Part model, mm, in its own coordinate system. Round coordinates to 2 decimals unless told otherwise and drop trailing zeros. Loops run counter-clockwise (first coordinate to the right, second up) from the corner with the lowest first, then second, coordinate; pieces in that order, holes last. Notation, with made-up numbers: M 3.5,-3 L 47.5,-3 A36 cw 47.5,36 Z; hole C 52,85.25 d10. An arc over 180 degrees is marked long. Put each result on its own line as item: value. Start each with the question number.
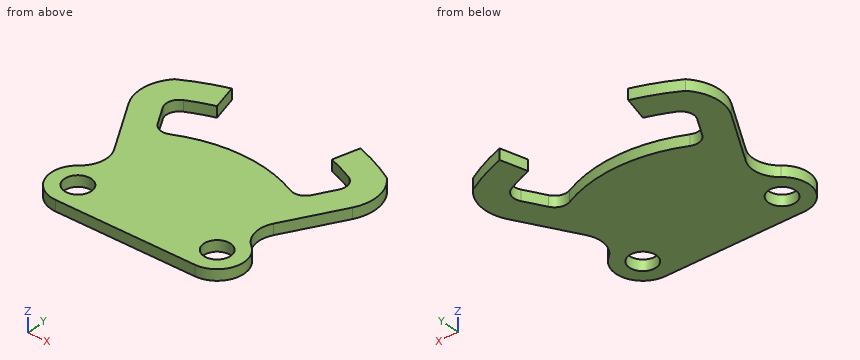
```python
from build123d import *

# Parameters (mm, degrees)
CROQUIS1_R              = 12.5
SALIENTE_EXTRUIR3_DEPTH = 10


with BuildPart() as part:
    # Croquis1 → Saliente-Extruir3 (new body)
    with BuildSketch(Plane.XY):
        with BuildLine():
            Line((-65, 0), (65, 0))
            ThreePointArc((65, 0), (88.615469852, 16.795758191), (80.499762007, 44.615233308))
            ThreePointArc((80.499762007, 44.615233308), (71.445806296, 59.527813514), (74.34888892, 76.730466615))
            Line((74.34888892, 76.730466615), (104.34888892, 128.691990842))
            ThreePointArc((104.34888892, 128.691990842), (109.189179993, 152.050160185), (99.153741511, 173.690919579))
            ThreePointArc((99.153741511, 173.690919579), (80.034708306, 183.287875939), (60, 190.787840283))
            Line((60, 190.787840283), (53.522714622, 166.614282159))
            ThreePointArc((53.522714622, 166.614282159), (65.481747035, 162.287217011), (77.094946128, 157.103053062))
            ThreePointArc((77.094946128, 157.103053062), (83.288324785, 149.82485993), (82.200740382, 140.330272281))
            Line((82.200740382, 140.330272281), (71.673300788, 122.09621203))
            ThreePointArc((71.673300788, 122.09621203), (64.832856812, 116.63391364), (56.102320229, 117.271180027))
            ThreePointArc((56.102320229, 117.271180027), (0, 130), (-56.102320229, 117.271180027))
            ThreePointArc((-56.102320229, 117.271180027), (-64.832856812, 116.63391364), (-71.673300788, 122.09621203))
            Line((-71.673300788, 122.09621203), (-82.200740382, 140.330272281))
            ThreePointArc((-82.200740382, 140.330272281), (-83.288324785, 149.82485993), (-77.094946128, 157.103053062))
            ThreePointArc((-77.094946128, 157.103053062), (-65.481747035, 162.287217011), (-53.522714622, 166.614282159))
            Line((-53.522714622, 166.614282159), (-60, 190.787840283))
            ThreePointArc((-60, 190.787840283), (-80.034708306, 183.287875939), (-99.153741511, 173.690919579))
            ThreePointArc((-99.153741511, 173.690919579), (-109.189179993, 152.050160185), (-104.34888892, 128.691990842))
            Line((-104.34888892, 128.691990842), (-74.34888892, 76.730466615))
            ThreePointArc((-74.34888892, 76.730466615), (-71.445806296, 59.527813514), (-80.499762007, 44.615233308))
            ThreePointArc((-80.499762007, 44.615233308), (-88.615469852, 16.795758191), (-65, 0))
        make_face()
        with Locations((65, 25)):
            Circle(CROQUIS1_R, mode=Mode.SUBTRACT)
        with Locations(Location((-65, 25, 0), (0, 0, 180))):
            Circle(CROQUIS1_R, mode=Mode.SUBTRACT)
    extrude(amount=SALIENTE_EXTRUIR3_DEPTH)


solid = part.part
```
1. Drop flat-ended pins along their axis: pin 1 (4 mm diameter, centred on x = -2.5, z = 2, fed in from +Y); pin 2 (1.5 mm diameter, centred on y = 69, z = 7.5, fed in from +X); pin 3 (1.5 mm diameter, centred on y = 53, z = 8.5, fed in from +X). Give the stop position or say it passes through.
2. Cut at C-C, the plane y = 135. Give the cut face in (x, z), and give its area (3 significant figures).
3. Wall check: L1, parallel to X at y = 33.5, z = 7.5; L2, parallel to Y at x = 65, z = 6.5; L3, parallel to X at y = 118, z = 5.25. Give the ranges that are in metal, low to high.
4. Cut at B-B, the plane z = 5.25. Give the cut face in (x, y).
5. Cut at D-D, the plane x = 94.5. Give the cut face in (y, z), and give its area (3 significant figures).
6. Cut at A-A, the plane y = 25. Give the cut face in (x, z), and give its area (3 significant figures).
Results list:
1. pin 1: stops at y = 130
1. pin 2: stops at x = 71.62
1. pin 3: stops at x = 74.06
2. outline: M -107.26,0 L -79.12,0 L -79.12,10 L -107.26,10 Z; M 79.12,0 L 107.26,0 L 107.26,10 L 79.12,10 Z
2. area: 563 mm^2
3. L1: x = -88.51 to -74.17, -55.83 to 55.83, 74.17 to 88.51
3. L2: y = 0 to 12.5, 37.5 to 116.69, 162.48 to 189.14
3. L3: x = -98.18 to -67.77, -54.55 to 54.55, 67.77 to 98.18
4. outline: M -104.35,128.69 L -74.35,76.73 A25 cw -80.5,44.62 A25 ccw -65,0 L 65,0 A25 ccw 80.5,44.62 A25 cw 74.35,76.73 L 104.35,128.69 A38 ccw 99.15,173.69 A200 ccw 60,190.79 L 53.52,166.61 A175 cw 77.09,157.1 A12 cw 82.2,140.33 L 71.67,122.1 A12 cw 56.1,117.27 A130 ccw -56.1,117.27 A12 cw -71.67,122.1 L -82.2,140.33 A12 cw -77.09,157.1 A175 cw -53.52,166.61 L -60,190.79 A200 ccw -99.15,173.69 A38 ccw Z; hole C -65,25 d25; hole C 65,25 d25
5. outline: M 111.63,0 L 176.27,0 L 176.27,10 L 111.63,10 Z
5. area: 646 mm^2
6. outline: M -90,0 L -77.5,0 L -77.5,10 L -90,10 Z; M -52.5,0 L 52.5,0 L 52.5,10 L -52.5,10 Z; M 77.5,0 L 90,0 L 90,10 L 77.5,10 Z
6. area: 1,300 mm^2
